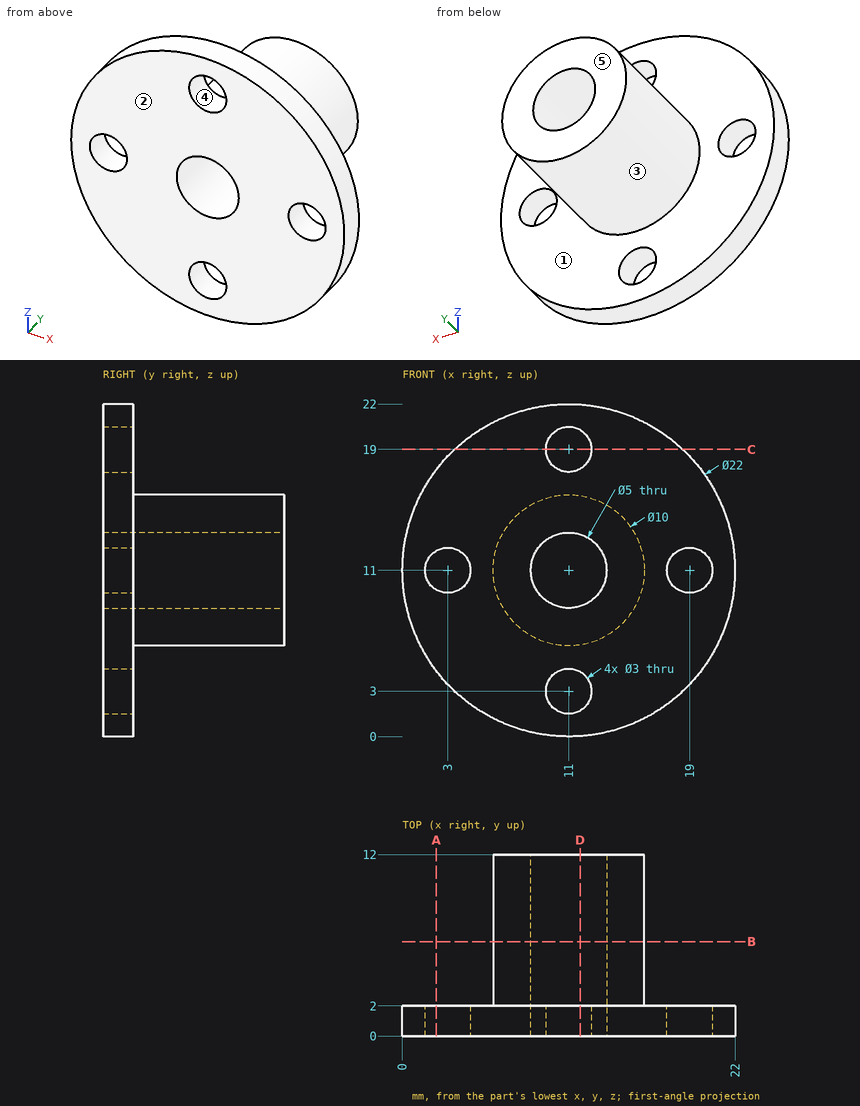
Here's the drawing with two shaded views (mm, measured from the low corner). I have some questions. A direction names the side the tool comes from. Give positions to 0.01 mm unless a question says otherwise; leave off trailing zeros. Loops run counter-clockwise (first coordinate to the right, second up) from the corner with the lowest first, then second, coordinate; pieces in that order, holes last. Notation, with made-up numbers: (-11, -31) - (43, -31) arc R20 ccw to (43, -8) - close; hole circle Ø7 at (61, 83). An arc over 180 degrees is marked (long way). Answer in a Markdown table with one row per item. Add a question column.
Q1. If we section it at C-C (z = 19): List the corners of the cut face in (x, y) for me.
Q2. For pin 1 (4 mm diameter, centred on x = 3, z = 11, fed in from +Y); pin 2 (3 mm diameter, centred on x = 8.5, y = 7, fed in from -Z); pin 3 (5 mm diameter, centred on x = 6, y = 7.5, fed in from +Z); pin 4 (4.5 mm diameter, centred on x = 11, z = 11, fed in from -Y), each with a flat end and sliding along its axis, tell me the tip position at first contact or that it passes through.
Q3. Please list where these lines run through material, in increasing order: L1, parallel to Z at x = 11, y = 6; L2, parallel to Y at x = 17.5, z = 14.75; L3, parallel to Z at x = 3, y = 1.15. Write a range as from..to.
Q4. If we section it at A-A (x = 2.25): List the corners of the cut face in (y, z) for me.
Q5. If we section it at B-B (y = 6.25): List the corners of the cut face in (x, z) for me, plus the area to 3 significant figures.
Q6. We'd pull the mould along X, two halves only. Please class the marked faces 3, 4 and 5: +X half, -X half, draft (parallel to the pull), parting line (faces both ways), or undercut.
Q7. Which directions (+Z, -Z, +X, -X, +Y, -Y) give clear straight access to the entire face, cutting with the end or side of a thin tool? Please do the marked faces 1 and 2.
Q8. If we section it at D-D (x = 11.75): List the corners of the cut face in (y, z) for me, plus the area to 3 significant figures.
The answers:
| question | item | result |
|---|---|---|
| 1 | outline | (3.45, 0) - (9.5, 0) - (9.5, 2) - (3.45, 2) - close; (12.5, 0) - (18.55, 0) - (18.55, 2) - (12.5, 2) - close |
| 2 | pin 1 | stops at y = 2 |
| 2 | pin 2 | stops at z = 6.1 |
| 2 | pin 3 | stops at z = 15.33 |
| 2 | pin 4 | passes through |
| 3 | L1 | z = 6..8.5, 13.5..16 |
| 3 | L2 | y = 0..2 |
| 3 | L3 | z = 3.45..9.5, 12.5..18.55 |
| 4 | outline | (0, 4.33) - (2, 4.33) - (2, 9.7) - (0, 9.7) - close; (0, 12.3) - (2, 12.3) - (2, 17.67) - (0, 17.67) - close |
| 5 | outline | circle Ø10 at (11, 11); hole circle Ø5 at (11, 11) |
| 5 | area | 58.9 mm^2 |
| 6 | face 3 | parting line |
| 6 | face 4 | undercut |
| 6 | face 5 | draft |
| 7 | face 1 | +Y |
| 7 | face 2 | +Z, -Z, +X, -X, -Y |
| 8 | outline | (0, 0.03) - (2, 0.03) - (2, 1.7) - (0, 1.7) - close; (0, 4.3) - (2, 4.3) - (2, 6.06) - (12, 6.06) - (12, 8.62) - (0, 8.62) - close; (0, 13.38) - (12, 13.38) - (12, 15.94) - (2, 15.94) - (2, 17.7) - (0, 17.7) - close; (0, 20.3) - (2, 20.3) - (2, 21.97) - (0, 21.97) - close |
| 8 | area | 75.1 mm^2 |
